Can you work these out from the drawing? Everything is in mm from the part's minimum corner. Round coordinates to 2 decimals unless told otherwise and drop trailing zeros. Write each loop counter-clockwise with the first axis right and the second up, starting at its lowest first coordinate (ties: lowest second). Pieces come first, ordered by that corner, then holes. Notation, with made-up numbers: M 34.25,-30 L 62.25,-30 A18 ccw 62.25,-18 Z; hole C -1.5,-9 d11. An arc over 180 degrees is marked long. Use one line per item in the form item = value. Start each with the question number.
Q1. I want a section at B-B on x = 12.7. List the corners of the cut face in (y, z) for me.
Q2. I need wall thicknesses on line 1 along Y through (x, z) = (12.7, 32); line 2 along Y through (x, z) = (63, 11); line 3 along X through (y, z) = (38.1, 26). Which ranges of each line are inside material? Lowest first, please. Write a range as from..to.
Q3. I want a section at A-A on y = 38.1. List the corners of the cut face in (x, z) for me.
Q4. I want a section at D-D on z = 43.5. State how many separate pieces and enclosed holes the cut face has, and give its area (3 significant figures).
Q5. We'd pull the mould along X, two halves only. Please class the marked faces 1, 2 and 3: +X half, -X half, draft (parallel to the pull), parting line (faces both ways), or undercut.
Q6. I'm going to push a flat-ended pin straight in: pin 1 Ø7.5 at (x, y) = (114.3, 63.5) entering from +Z. Where does the tip first touch, or does it pass through?
Q7. I want a section at C-C on x = 63.5. List the corners of the cut face in (y, z) for me.
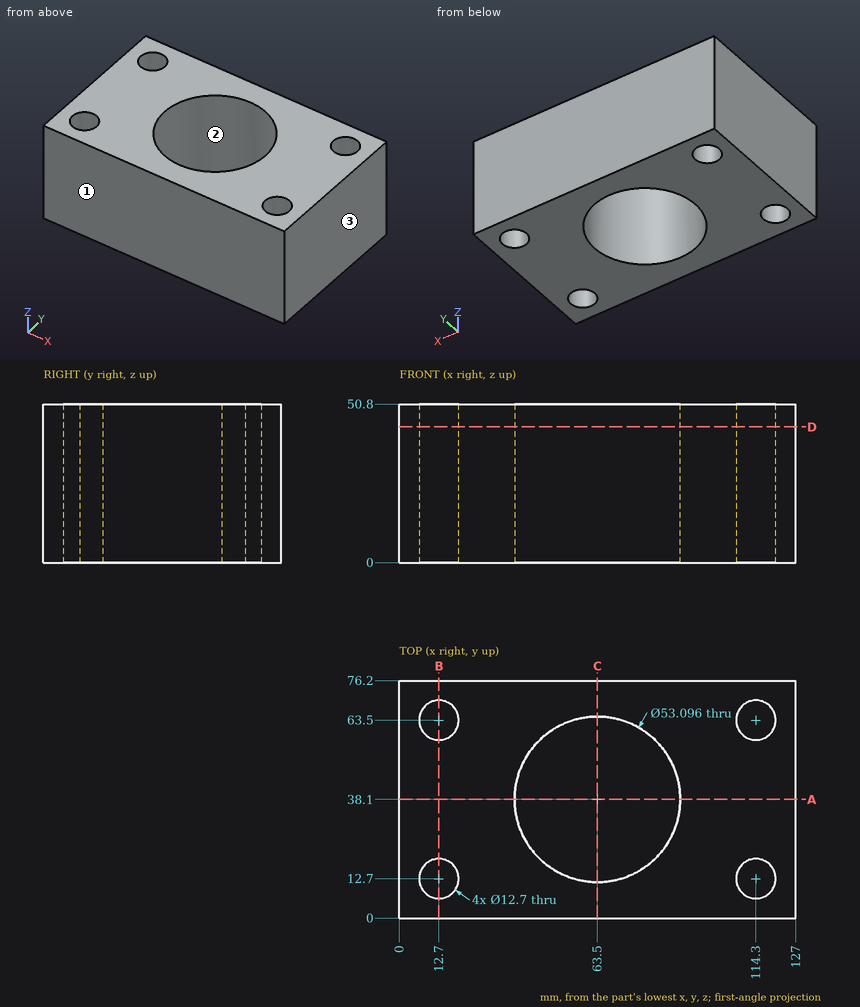
Reported:
q1.outline = M 0,0 L 6.35,0 L 6.35,50.8 L 0,50.8 Z; M 19.05,0 L 57.15,0 L 57.15,50.8 L 19.05,50.8 Z; M 69.85,0 L 76.2,0 L 76.2,50.8 L 69.85,50.8 Z
q2.line_1 = 0..6.35, 19.05..57.15, 69.85..76.2
q2.line_2 = 0..11.56, 64.64..76.2
q2.line_3 = 0..36.95, 90.05..127
q3.outline = M 0,0 L 36.95,0 L 36.95,50.8 L 0,50.8 Z; M 90.05,0 L 127,0 L 127,50.8 L 90.05,50.8 Z
q4.separate_pieces = 1
q4.enclosed_holes = 5
q4.area = 6,960 mm^2
q5.face_1 = draft
q5.face_2 = undercut
q5.face_3 = +X half
q6.pin_1 = through
q7.outline = M 0,0 L 11.55,0 L 11.55,50.8 L 0,50.8 Z; M 64.65,0 L 76.2,0 L 76.2,50.8 L 64.65,50.8 Z
